```python
from build123d import *

# Parameters (mm, degrees)
BOSS_EXTRUDE1_DEPTH = 1.5
SKETCH3_R           = 10.5
BOSS_EXTRUDE2_DEPTH = 1
FILLET1_R           = 0.5
BOSS_EXTRUDE3_START = 4
SKETCH4_R           = 10.5
BOSS_EXTRUDE3_DEPTH = 4
FILLET2_R           = 0.5
SKETCH6_R           = 4
BOSS_EXTRUDE4_DEPTH = 8
SKETCH7_R           = 5.5
BOSS_EXTRUDE5_DEPTH = 10


with BuildPart() as part:
    # Sketch1 → Boss-Extrude1 (new, symmetric)
    with BuildSketch(Plane.XY):
        with BuildLine():
            ThreePointArc((8.079170849, 18.840833272), (7.548253676, 19.059744658), (7.011412938, 19.263698726))
            ThreePointArc((7.011412938, 19.263698726), (6.469069926, 19.452535421), (5.92165025, 19.62610655))
            ThreePointArc((5.92165025, 19.62610655), (4.769916061, 18.460076292), (3.92920603, 17.053191489))
            ThreePointArc((3.92920603, 17.053191489), (0, 14.5), (-3.92920603, 17.053191489))
            ThreePointArc((-3.92920603, 17.053191489), (-4.769916061, 18.460076292), (-5.92165025, 19.62610655))
            ThreePointArc((-5.92165025, 19.62610655), (-6.469069926, 19.452535421), (-7.011412938, 19.263698726))
            ThreePointArc((-7.011412938, 19.263698726), (-7.548253676, 19.059744658), (-8.079170849, 18.840833272))
            ThreePointArc((-8.079170849, 18.840833272), (-8.211940621, 17.207281806), (-7.95163375, 15.58914753))
            ThreePointArc((-7.95163375, 15.58914753), (-9.32042034, 11.107644425), (-13.97152664, 10.537857626))
            ThreePointArc((-13.97152664, 10.537857626), (-15.519876007, 11.07519592), (-17.151665385, 11.228106453))
            ThreePointArc((-17.151665385, 11.228106453), (-17.459443815, 10.743268669), (-17.753520778, 10.25))
            ThreePointArc((-17.753520778, 10.25), (-18.033665494, 9.748687545), (-18.299658117, 9.239724714))
            ThreePointArc((-18.299658117, 9.239724714), (-17.351339022, 7.903008926), (-16.111815726, 6.830768187))
            ThreePointArc((-16.111815726, 6.830768187), (-14.279712419, 2.517898576), (-17.476414659, -0.908256936))
            ThreePointArc((-17.476414659, -0.908256936), (-19.007913485, -1.491891711), (-20.356225667, -2.423649439))
            ThreePointArc((-20.356225667, -2.423649439), (-20.280349902, -2.992892892), (-20.188558937, -3.559787642))
            ThreePointArc((-20.188558937, -3.559787642), (-20.080924805, -4.123888815), (-19.957531975, -4.684753727))
            ThreePointArc((-19.957531975, -4.684753727), (-18.371853055, -5.099169663), (-16.73310006, -5.123803506))
            ThreePointArc((-16.73310006, -5.123803506), (-12.557368355, -7.25), (-12.80389403, -11.929387983))
            ThreePointArc((-12.80389403, -11.929387983), (-13.601936994, -13.360906629), (-14.035881725, -14.941352824))
            ThreePointArc((-14.035881725, -14.941352824), (-13.611854879, -15.328646605), (-13.177145999, -15.703911084))
            ThreePointArc((-13.177145999, -15.703911084), (-12.732096226, -16.066851767), (-12.277054818, -16.417183833))
            ThreePointArc((-12.277054818, -16.417183833), (-10.795972864, -15.715390096), (-9.524780909, -14.680890594))
            ThreePointArc((-9.524780909, -14.680890594), (-4.959292078, -13.625543001), (-2.140289085, -17.368625813))
            ThreePointArc((-2.140289085, -17.368625813), (-1.831463015, -18.978204846), (-1.147992733, -20.467831167))
            ThreePointArc((-1.147992733, -20.467831167), (-0.574221679, -20.491956214), (0, -20.5))
            ThreePointArc((0, -20.5), (0.574221679, -20.491956214), (1.147992733, -20.467831167))
            ThreePointArc((1.147992733, -20.467831167), (1.831463015, -18.978204846), (2.140289085, -17.368625813))
            ThreePointArc((2.140289085, -17.368625813), (4.959292078, -13.625543001), (9.524780909, -14.680890594))
            ThreePointArc((9.524780909, -14.680890594), (10.795972864, -15.715390096), (12.277054818, -16.417183833))
            ThreePointArc((12.277054818, -16.417183833), (12.732096226, -16.066851767), (13.177145999, -15.703911084))
            ThreePointArc((13.177145999, -15.703911084), (13.611854879, -15.328646605), (14.035881725, -14.941352824))
            ThreePointArc((14.035881725, -14.941352824), (13.601936994, -13.360906629), (12.80389403, -11.929387983))
            ThreePointArc((12.80389403, -11.929387983), (12.557368355, -7.25), (16.73310006, -5.123803506))
            ThreePointArc((16.73310006, -5.123803506), (18.371853055, -5.099169663), (19.957531975, -4.684753727))
            ThreePointArc((19.957531975, -4.684753727), (20.080924805, -4.123888815), (20.188558937, -3.559787642))
            ThreePointArc((20.188558937, -3.559787642), (20.280349902, -2.992892892), (20.356225667, -2.423649439))
            ThreePointArc((20.356225667, -2.423649439), (19.007913485, -1.491891711), (17.476414659, -0.908256936))
            ThreePointArc((17.476414659, -0.908256936), (14.279712419, 2.517898576), (16.111815726, 6.830768187))
            ThreePointArc((16.111815726, 6.830768187), (17.351339022, 7.903008926), (18.299658117, 9.239724714))
            ThreePointArc((18.299658117, 9.239724714), (18.033665494, 9.748687545), (17.753520778, 10.25))
            ThreePointArc((17.753520778, 10.25), (17.459443815, 10.743268669), (17.151665385, 11.228106453))
            ThreePointArc((17.151665385, 11.228106453), (15.519876007, 11.07519592), (13.97152664, 10.537857626))
            ThreePointArc((13.97152664, 10.537857626), (9.32042034, 11.107644425), (7.95163375, 15.58914753))
            ThreePointArc((7.95163375, 15.58914753), (8.211940621, 17.207281806), (8.079170849, 18.840833272))
        make_face()
    extrude(amount=BOSS_EXTRUDE1_DEPTH, both=True)

    # Sketch2 → Cut-Revolve2 (revolve, cut)
    with BuildSketch(Plane(origin=(0, 0, 0), x_dir=(0, 0, -1), z_dir=(1, 0, 0))):
        with BuildLine():
            Line((-1.5, -17.5), (-1.5, -20.5))
            Line((-1.5, -20.5), (-1, -20.5))
            ThreePointArc((-1, -20.5), (-1.374143795, -19.020690633), (-1.5, -17.5))
        make_face()
    cut_revolve2 = revolve(axis=Axis((0, 0, 0), (0, 0, 1)), mode=Mode.SUBTRACT)

    # Mirror1: Cut-Revolve2 across plane
    add(cut_revolve2.mirror(Plane.XY), mode=Mode.SUBTRACT)

    # Sketch3 → Boss-Extrude2 (add)
    with BuildSketch(Plane.XY.offset(1.5)):
        Circle(SKETCH3_R)
    extrude(amount=BOSS_EXTRUDE2_DEPTH)

    # Fillet1
    fillet1_edges = [part.edges().sort_by_distance(p)[0] for p in [
        (-10.5, 0, 1.5),
    ]]
    fillet(fillet1_edges, radius=FILLET1_R)

    # Sketch4 → Boss-Extrude3 (add)
    with BuildSketch(Plane(origin=(0, 0, -1.5), x_dir=(-1, 0, 0), z_dir=(0, 0, -1)).offset(BOSS_EXTRUDE3_START)):
        with Locations(Location((0, 0, 0), (0, 0, 180))):
            Circle(SKETCH4_R)
    extrude(amount=-BOSS_EXTRUDE3_DEPTH)

    # Fillet2
    fillet2_edges = [part.edges().sort_by_distance(p)[0] for p in [
        (-10.5, 0, -1.5),
    ]]
    fillet(fillet2_edges, radius=FILLET2_R)

    # Sketch6 → Boss-Extrude4 (add)
    with BuildSketch(Plane.XY.offset(2.5)):
        Circle(SKETCH6_R)
    extrude(amount=BOSS_EXTRUDE4_DEPTH)

    # Sketch7 → Boss-Extrude5 (add)
    with BuildSketch(Plane(origin=(0, 0, -5.5), x_dir=(-1, 0, 0), z_dir=(0, 0, -1))):
        Circle(SKETCH7_R)
    extrude(amount=BOSS_EXTRUDE5_DEPTH)


solid = part.part
```
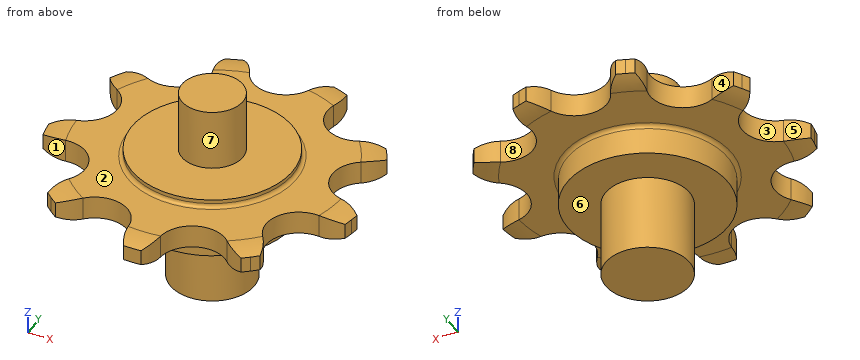
Here's how the part is built. I have some questions about the finished solid (model axes, mm). Face numbers are marked on the shaded views. A direction names the side the tool comes from. Give positions to 0.01 mm unless a question says otherwise; leave off trailing zeros. Write each loop counter-clockwise with the first axis right and the second up, starting at its lowest first coordinate (ties: lowest second). Pieces come first, ordered by that corner, then holes. Notation, with made-up numbers: (69.5, 60) -> (81.5, 60) arc R21 ccw to (81.5, 86) -> close; hole circle Ø3 at (76.5, 4.25). An arc over 180 degrees is marked (long way). Write each question's results on one line, items separated by ' | '.
Item 1: On a 3-axis mill with a long thin cutter (end or side, diameter ignored), from which of +Z, -Z, +X, -X, +Y, -Y can I reach the whole of each face in a straight line? I mean the marked faces 4, 5, 6, 7 and 8. Say none if no direction works.
Output:
face 4: +Z, -Z, +Y | face 5: +Z, -Z, -X | face 6: -Z | face 7: +Z | face 8: +Z, -Z
Item 2: Suppose I cut it at A-A on x = 0. Write out the boundary of the cut face in (y, z), plus the area to 3 significant figures.
Output:
outline: (-20.5, -1) arc R9.25 ccw to (-17.5, -1.5) -> (-11, -1.5) arc R0.5 cw to (-10.5, -2) -> (-10.5, -5.5) -> (-5.5, -5.5) -> (-5.5, -15.5) -> (5.5, -15.5) -> (5.5, -5.5) -> (10.5, -5.5) -> (10.5, -2) arc R0.5 cw to (11, -1.5) -> (14.5, -1.5) -> (14.5, 1.5) -> (11, 1.5) arc R0.5 cw to (10.5, 2) -> (10.5, 2.5) -> (4, 2.5) -> (4, 10.5) -> (-4, 10.5) -> (-4, 2.5) -> (-10.5, 2.5) -> (-10.5, 2) arc R0.5 cw to (-11, 1.5) -> (-17.5, 1.5) arc R9.25 ccw to (-20.5, 1) -> close | area: 383 mm^2
Item 3: For pin 1 Ø3 at (x, z) = (15.5, 4.5) entering from -Y; pin 2 Ø1 at (y, z) = (4, 7) entering from +X; pin 3 Ø8 at (y, z) = (14, -0.5) entering from -X; pin 4 Ø1 at (x, y) = (-5.5, -10) entering from -Z, each with a flat end and sliding along its axis, tell me the tip position at first contact or that it passes through.
Output:
pin 1: passes through | pin 2: stops at x = 1.94 | pin 3: stops at x = -17.9 | pin 4: stops at z = -1.51
Item 4: Suppose I cut it at B-B on z = 6. Write out the boundary of the cut face in (x, y).
Output:
outline: circle Ø8 at (0, 0)
Item 5: Suppose I cut it at D-D on y = -14. Give the number of separate pieces and of enclosed holes in the cut face, plus the area to 3 significant figures.
Output:
separate pieces: 3 | enclosed holes: 0 | area: 54.9 mm^2
Item 6: Suppose I cut it at C-C on y = 0. Write out the boundary of the cut face in (x, z), plus the area to 3 significant figures.
Output:
outline: (-15.72, -1.5) -> (-11, -1.5) arc R0.5 cw to (-10.5, -2) -> (-10.5, -5.5) -> (-5.5, -5.5) -> (-5.5, -15.5) -> (5.5, -15.5) -> (5.5, -5.5) -> (10.5, -5.5) -> (10.5, -2) arc R0.5 cw to (11, -1.5) -> (15.72, -1.5) -> (15.72, 1.5) -> (11, 1.5) arc R0.5 cw to (10.5, 2) -> (10.5, 2.5) -> (4, 2.5) -> (4, 10.5) -> (-4, 10.5) -> (-4, 2.5) -> (-10.5, 2.5) -> (-10.5, 2) arc R0.5 cw to (-11, 1.5) -> (-15.72, 1.5) -> close | area: 374 mm^2
Item 7: If I drill on L1, parallel to Z at x = -11.5, y = 3; L2, parallel to Z at x = 6, y = -6.5; L3, parallel to X at y = -2, z = 1.75, over which ranges is the centre line in solid material (lowest first)?
Output:
L1: z = -1.5 to 1.5 | L2: z = -5.5 to 2.5 | L3: x = -10.38 to 10.38
Item 8: We'd pull the mould along X, two halves only. Please class the marked faces 1, 2 and 3: pulls with the +X half, pulls with the -X half, needs draft (parallel to the pull), parting line crosses it, or undercut.
Output:
face 1: undercut | face 2: needs draft | face 3: pulls with the -X half
